For this review, take the finished solid that the model builds, in its own axes (mm). Coordinates: 2 decimals unless noted, no trailing zeros. Order: outer loops, then holes, each group sorted by start corner. A loop starts at its lowest first (then second) coordinate and runs counter-clockwise, first axis right, second up. Notation, with made-up numbers: (-25.5, 33) -> (-8.5, 33) arc R10 ccw to (-8.5, 51) -> close; hole circle Ø6 at (7.25, 86.25). An arc over 180 degrees is marked (long way). Write item = value, one per line. Start each with the question number.
1) Insertion check: pin 1 Ø0.5 at (x, y) = (-2.5, 1.5) entering from -Z; pin 2 Ø0.5 at (x, y) = (3, 0) entering from +Z; pin 3 Ø5 at (x, z) = (3.5, 24) entering from +Y; pin 4 Ø1.5 at (x, y) = (-1, -4.5) entering from -Z. Each pin has a flat end and moves straight along its axis. Give the tip position at first contact, or say it passes through.
2) Draft analysis for pull direction Z (two halves, no side actions). For faces 1 (the face through (3.174, 1, 19.839)), 2 (the face through (-1.5, 2.8, 39)), state which applies: +Z half, -Z half, draft (parallel to the pull), parting line (faces both ways), or undercut.
3) Consider section A-A on x = 4.5. Give the boundary of the cut face in (y, z).
4) Wall thickness on probe 1 along Y at (x, z) = (0, 38.65); probe 2 along Z at (x, y) = (-2.75, 5); probe 3 along Y at (x, z) = (1.75, 26.5): over which ranges is each line inside the solid? List them lowest first. Write a range as [from, to].
from build123d import *

# Parameters (mm, degrees)
SKETCH1_R          = 3.32812519
BASE_EXTRUDE_DEPTH = 35
LPATTERN1_COUNT    = 26
LPATTERN1_PITCH    = 1.249999972
SKETCH7_W          = 6.500000134
SKETCH7_H          = 8.00000038
CUT_EXTRUDE2_DEPTH = 4.00000019


with BuildPart() as part:
    # Sketch1 → Base-Extrude (new body)
    with BuildSketch(Plane.XY):
        Circle(SKETCH1_R)
    extrude(amount=BASE_EXTRUDE_DEPTH)

    # Boss-Sweep1: sweep along a path in Sketch4
    with BuildLine(Plane(origin=(0, 0, 0.5), x_dir=(-1, 0, 0), z_dir=(0, 0, -1))) as boss_sweep1_path:
        CenterArc((0, 0), 3.32812519, 0, 360)
    # Sketch2 → Boss-Sweep1 (sweep)
    with BuildSketch(Plane(origin=(0, 0, 0), x_dir=(1, 0, 0), z_dir=(0, 1, 0))):
        Polygon((3.32812519, 0), (4.00000019, -0.387907212), (4.00000019, -0.544157209), (3.32812519, -0.932064421), align=None)
    boss_sweep1 = sweep(path=boss_sweep1_path.line)

    # LPattern1: Boss-Sweep1 ×26
    with Locations(*[(0, 0, i * LPATTERN1_PITCH) for i in range(1, LPATTERN1_COUNT)]):
        add(boss_sweep1)

    # Sketch7 → Boss-Revolve2 (revolve)
    with BuildSketch(Plane(origin=(0, 0, 0), x_dir=(1, 0, 0), z_dir=(0, 1, 0))):
        with Locations((3.250000067, -39.00000019)):
            Rectangle(SKETCH7_W, SKETCH7_H)
    revolve(axis=Axis((0, 0, 0), (0, 0, 1)))

    # Sketch8 → Cut-Extrude2 (cut)
    with BuildSketch(Plane.XY.offset(43.00000038)):
        Polygon((-1.697949218, 3.000000026), (1.697949218, 3.000000026), (3.430000041, 0), (1.697949218, -3.000000026), (-1.697949218, -3.000000026), (-3.430000041, 0), align=None)
    extrude(amount=-CUT_EXTRUDE2_DEPTH, mode=Mode.SUBTRACT)

    # Sketch9 → Cut-Revolve1 (revolve, cut)
    with BuildSketch(Plane(origin=(0, 0, 0), x_dir=(1, 0, 0), z_dir=(0, 1, 0))):
        Polygon((0, -39.00000019), (3.000000026, -39.00000019), (3.000000026, -38.20000021), (0, -37.396152626), align=None)
    revolve(axis=Axis((0, 0, 0), (0, 0, 1)), mode=Mode.SUBTRACT)


solid = part.part
Answer sheet:
q1.pin_1 = 0
q1.pin_2 = 39
q1.pin_3 = 3.87
q1.pin_4 = 0.31
q2.face_1 = undercut
q2.face_2 = +Z half
q3.outline = (-4.69, 35) -> (4.69, 35) -> (4.69, 43) -> (-4.69, 43) -> close
q4.probe_1 = [-6.5, -3], [3, 6.5]
q4.probe_2 = [35, 43]
q4.probe_3 = [-3.33, 3.33]
